The model under review builds one solid part; all positions refer to its coordinate system, in mm. Coordinates: 2 decimals unless noted, no trailing zeros. Order: outer loops, then holes, each group sorted by start corner. A loop starts at its lowest first (then second) coordinate and runs counter-clockwise, first axis right, second up.
Autodesk Fusion 360 part; units mm, degrees
cylinder "CylinderPrimitive1" add diameter 23.8 height 4 placed x (1, 0, 0) y (0, 0, -1) z (0, 1, 0) at (0, 0, 0)
hole "Hole1" at (0, 4, 0) direction (0, -1, 0) diameter 6.4 end through all countersink diameter 12.6 countersink angle 90
chamfer "Chamfer1" distance 0.5 angle 45 2 edges at (-11.0947, 4, 4.3032) (-11.0947, 0, -4.3032)
sketch "Sketch4" plane through (0, 0, 0) normal (0, 1, 0) x (1, 0, 0)
  circle A0 centre (0, 0) radius 8.5 construction
  point P0 (-8.5, 0)
  dimension "d9" = 17
hole "Hole2" at (-8.5, 0, 0) direction (0, 1, 0) diameter 2 end through all
(1) Draft analysis for pull direction X (two halves, no side actions). For faces 1 (the face through (1.947, 0.444, -2.539)), 2 (the face through (2.4, 0, 2.4)), 3 (the face through (-8.771, 2.021, -8.043)), state which applies: released by +X, released by -X, zero draft, split by the parting line, or undercut.
A:
face 1: undercut
face 2: zero draft
face 3: split by the parting line
(2) We need section C-C, the plane y = 2.05. Write out the cut boundary in (x, z).
A:
outline: circle Ø23.8 at (0, 0); hole circle Ø2 at (-8.5, 0); hole circle Ø8.7 at (0, 0)
(3) We need section A-A, the plane z = 0. Write out the cut boundary in (x, y), and give its area (3 significant figures).
A:
outline: (-11.9, 0.5) - (-11.4, 0) - (-9.5, 0) - (-9.5, 4) - (-11.4, 4) - (-11.9, 3.5) - close; (-7.5, 0) - (-3.2, 0) - (-3.2, 0.9) - (-6.3, 4) - (-7.5, 4) - close; (3.2, 0) - (11.4, 0) - (11.9, 0.5) - (11.9, 3.5) - (11.4, 4) - (6.3, 4) - (3.2, 0.9) - close
area: 51.5 mm2
(4) Wall thickness on probe 1 along Z at (x, y) = (0, 0.55); probe 2 along X at (y, z) = (0.6, 0); probe 3 along X at (y, z) = (3.05, 0): over which ranges is each line inside the solid? List them lowest first.
A:
probe 1: z = -11.9 to -3.2, 3.2 to 11.9
probe 2: x = -11.9 to -9.5, -7.5 to -3.2, 3.2 to 11.9
probe 3: x = -11.9 to -9.5, -7.5 to -5.35, 5.35 to 11.9
(5) For pin 1 Ø3 at (x, z) = (0, -2) entering from +Y; pin 2 Ø8.5 at (x, z) = (0, 0) entering from +Y; pin 3 Ø1.5 at (y, z) = (3.5, 8.5) entering from -X, all flat-tipped, find the tip position at first contact; note any pin that passes through.
A:
pin 1: stops at y = 1.2
pin 2: stops at y = 1.95
pin 3: stops at x = -9.03
(6) We need section B-B, the plane x = 0. Write out the cut boundary in (y, z).
A:
outline: (0, -11.4) - (0.5, -11.9) - (3.5, -11.9) - (4, -11.4) - (4, -6.3) - (0.9, -3.2) - (0, -3.2) - close; (0, 3.2) - (0.9, 3.2) - (4, 6.3) - (4, 11.4) - (3.5, 11.9) - (0.5, 11.9) - (0, 11.4) - close
